from build123d import *

# Parameters (mm, degrees)
ESQUISSE1_R                = 32.5
BOSS_EXTRU_1_DEPTH         = 15
ESQUISSE2_R                = 22.5
ENL_V_MAT_EXTRU_1_DEPTH    = 2.5
ESQUISSE3_R                = 6.5
ENL_V_MAT_EXTRU_2_DEPTH    = 48.631397208
TROUS_DE_CENTRAGE_6_0MM1_D = 6


with BuildPart() as part:
    # Esquisse1 → Boss.-Extru.1 (new body)
    with BuildSketch(Plane.XY):
        Circle(ESQUISSE1_R)
    extrude(amount=BOSS_EXTRU_1_DEPTH)

    # Esquisse2 → Enlèv. mat.-Extru.1 (cut)
    with BuildSketch(Plane.XY.offset(15)):
        Circle(ESQUISSE2_R)
    extrude(amount=-ENL_V_MAT_EXTRU_1_DEPTH, mode=Mode.SUBTRACT)

    # Esquisse3 → Enlèv. mat.-Extru.2 (cut, through all)
    with BuildSketch(Plane.XY.offset(12.5)):
        Circle(ESQUISSE3_R)
    extrude(amount=-ENL_V_MAT_EXTRU_2_DEPTH, mode=Mode.SUBTRACT)

    # Trous de centrage Ø6.0mm1 (through all)
    with Locations(Plane.XY.offset(15)):
        with Locations((0, -27.5), (-26.562960223, 7.11752374), (26.562960223, 7.11752374)):
            Hole(TROUS_DE_CENTRAGE_6_0MM1_D / 2)


solid = part.part
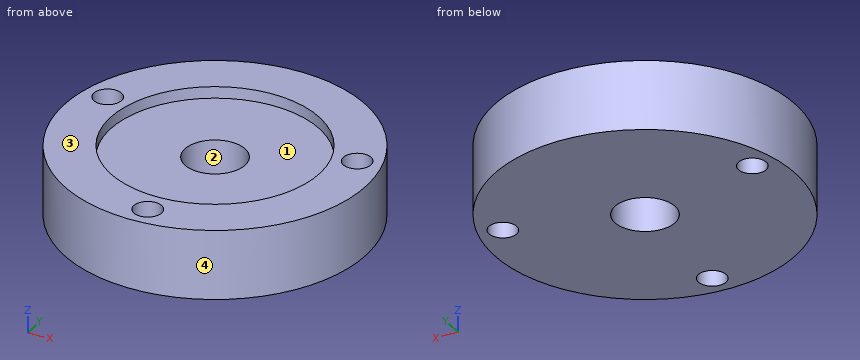
Source: CAD feature listing. Evaluate the final solid. Frame: model axes, mm. Face numbers are marked on the shaded views. Coordinates: 2 decimals unless noted, no trailing zeros. Write each loop counter-clockwise with the first axis right and the second up, starting at its lowest first coordinate (ties: lowest second). Pieces come first, ordered by that corner, then holes. Notation, with made-up numbers: M -9.5,16.25 L -5.5,16.25 A18 cw -5.5,41.25 Z; hole C 73.25,72.25 d7. An arc over 180 degrees is marked long. Use a Markdown table: item, result.
1) Section B-B, the plane y = 0. Output: boundary loops of the cut face in (x, z), then the cut area to 3 significant figures.
Conclusion:
| item | result |
|---|---|
| outline | M -32.5,0 L -6.5,0 L -6.5,12.5 L -22.5,12.5 L -22.5,15 L -32.5,15 Z; M 6.5,0 L 32.5,0 L 32.5,15 L 22.5,15 L 22.5,12.5 L 6.5,12.5 Z |
| area | 700 mm^2 |
2) Section D-D, the plane z = 2.5. Output: boundary loops of the cut face in (x, y).
Conclusion:
| item | result |
|---|---|
| outline | C 0,0 d65; hole C -26.56,7.12 d6; hole C 0,0 d13; hole C 0,-27.5 d6; hole C 26.56,7.12 d6 |
3) Ray query, L1, parallel to Y at x = 0, z = 3.75; L2, parallel to X at y = 8.5, z = 10; L3, parallel to Y at x = 0, z = 13.55. Return the intervals inside material, ascending.
Conclusion:
| item | result |
|---|---|
| L1 | y = -32.5 to -30.5, -24.5 to -6.5, 6.5 to 32.5 |
| L2 | x = -31.37 to -29.23, -23.9 to 23.9, 29.23 to 31.37 |
| L3 | y = -32.5 to -30.5, -24.5 to -22.5, 22.5 to 32.5 |
4) First-contact query: pin 1 Ø2 at (y, z) = (1, 4.5) entering from +X; pin 2 Ø5 at (x, y) = (6, 14) entering from +Z; pin 3 Ø5 at (y, z) = (-11, 5.5) entering from +X; pin 4 Ø1.5 at (y, z) = (3.5, 5) entering from -X. Flat tips, straight axial feed; report the tip coordinate or a pass-through.
Conclusion:
| item | result |
|---|---|
| pin 1 | stops at x = 32.5 |
| pin 2 | stops at z = 12.5 |
| pin 3 | stops at x = 31.37 |
| pin 4 | stops at x = -32.38 |
5) Mould query, pull axis X, two halves, no side actions, for the marked faces 1, 2, 3 and 4. Classes: pulls with the +X half, pulls with the -X half, needs draft (parallel to the pull), parting line crosses it, or undercut.
Conclusion:
| item | result |
|---|---|
| face 1 | undercut |
| face 2 | undercut |
| face 3 | needs draft |
| face 4 | parting line crosses it |
6) Section C-C, the plane y = 8. Output: boundary loops of the cut face in (x, z), then the cut area to 3 significant figures.
Conclusion:
| item | result |
|---|---|
| outline | M -31.5,0 L -29.43,0 L -29.43,15 L -31.5,15 Z; M -23.7,0 L 23.7,0 L 23.7,15 L 21.03,15 L 21.03,12.5 L -21.03,12.5 L -21.03,15 L -23.7,15 Z; M 29.43,0 L 31.5,0 L 31.5,15 L 29.43,15 Z |
| area | 668 mm^2 |
7) Section A-A, the plane x = 0. Output: boundary loops of the cut face in (y, z), then the cut area to 3 significant figures.
Conclusion:
| item | result |
|---|---|
| outline | M -32.5,0 L -30.5,0 L -30.5,15 L -32.5,15 Z; M -24.5,0 L -6.5,0 L -6.5,12.5 L -22.5,12.5 L -22.5,15 L -24.5,15 Z; M 6.5,0 L 32.5,0 L 32.5,15 L 22.5,15 L 22.5,12.5 L 6.5,12.5 Z |
| area | 610 mm^2 |
